from build123d import *

# Parameters (mm, degrees)
SKETCH_1_R          = 58.5
SKETCH_1_R_2        = 57.5
EXTRUDE_1_DEPTH     = 20
SKETCH_3_R          = 2
CUT_EXTRUDE_1_DEPTH = 71
SKETCH_4_R          = 2
CUT_EXTRUDE_2_DEPTH = 71


with BuildPart() as part:
    # 草图1 → 凸台-拉伸1 (new body)
    with BuildSketch(Plane(origin=(0, 0, 0), x_dir=(1, 0, 0), z_dir=(0, 1, 0))):
        with Locations(Location((0, 0, 0), (0, 0, 270))):
            Circle(SKETCH_1_R)
        with Locations(Location((0, 0, 0), (0, 0, 270))):
            Circle(SKETCH_1_R_2, mode=Mode.SUBTRACT)
    extrude(amount=EXTRUDE_1_DEPTH)

    # 草图3 → 切除-拉伸1 (cut)
    with BuildSketch(Plane(origin=(0, 0, 0), x_dir=(-0.12186934340515121, 0, -0.9925461516413215), z_dir=(0.9925461516413215, 0, -0.12186934340515121))):
        with Locations((0, 11)):
            Circle(SKETCH_3_R)
        with Locations((0, 4)):
            Circle(SKETCH_3_R)
    extrude(amount=-CUT_EXTRUDE_1_DEPTH, mode=Mode.SUBTRACT)

    # 草图4 → 切除-拉伸2 (cut)
    with BuildSketch(Plane(origin=(0, 0, 0), x_dir=(0.12186934340514427, 0, -0.9925461516413224), z_dir=(0.9925461516413224, 0, 0.12186934340514427))):
        with Locations((0, 11)):
            Circle(SKETCH_4_R)
        with Locations((0, 4)):
            Circle(SKETCH_4_R)
    extrude(amount=-CUT_EXTRUDE_2_DEPTH, mode=Mode.SUBTRACT)


solid = part.part
The listing builds one solid part. Answer for the finished solid, in the listing's coordinates (mm). Round coordinates to 2 decimals unless told otherwise and drop trailing zeros. Write each loop counter-clockwise with the first axis right and the second up, starting at its lowest first coordinate (ties: lowest second). Pieces come first, ordered by that corner, then holes. Notation, with made-up numbers: M 23.5,-22.5 L 82.5,-22.5 A20 ccw 82.5,15.5 Z; hole C 18,-9 d10. An arc over 180 degrees is marked long. Write each question's results on one line, items separated by ' | '. Start each with the question number.
(1) Determine the mould class of faces 1 (the flat face through (-39, 0, 43)), 2 (the cylindrical face through (-57.36, 12.35, 8.53)), 3 (the cylindrical face through (-57.656, 2.226, 6.149)), 4 (the flat face through (-39, 20, 43)) for opening direction Y: +Y half, -Y half, draft (parallel to the pull), parting line (faces both ways), or undercut.
(2) The part is cut by section A-A, the plane x = 0. Write down the section's boundary in (y, z), and give its area (3 significant figures).
(3) The part is cut by section B-B, the plane z = 0. Write down the section's boundary in (x, y).
(4) Each of these flat-tipped pins is pushed along its axis until it touches: P1, Ø2, axis at x = -44.5, y = 2.5, coming from the +Z side; P2, Ø8, axis at y = 10.5, z = -19.5, coming from the -X side; P3, Ø1, axis at x = -12, y = 14.5, coming from the +Z side. Where does it stop, or does it pass through?
(5) Find the intervals of material crossed by line 1 (X direction, y = 10.75, z = 0); line 2 (Z direction, x = 16, y = 1.5); line 3 (Z direction, x = -18, y = 7.5), in increasing order.
(6) The part is cut by section C-C, the plane y = 14.5. Write down the section's boundary in (x, z), and give its area (3 significant figures).
Worked answers:
1) face 1: -Y half | face 2: undercut | face 3: undercut | face 4: +Y half
2) outline: M 0,-58.5 L 20,-58.5 L 20,-57.5 L 0,-57.5 Z; M 0,57.5 L 20,57.5 L 20,58.5 L 0,58.5 Z | area: 40.0 mm²
3) outline: M -58.5,0 L -57.5,0 L -57.5,20 L -58.5,20 Z; M 57.5,0 L 58.5,0 L 58.5,20 L 57.5,20 Z
4) P1: stops at z = 39.12 | P2: stops at x = -56.41 | P3: stops at z = 57.36
5) line 1: x = -58.5 to -57.5, 57.5 to 58.5 | line 2: z = -56.27 to -55.23, 55.23 to 56.27 | line 3: z = -55.66 to -54.61, 54.61 to 55.66
6) outline: C 0,0 d117; hole C 0,0 d115 | area: 364 mm²
